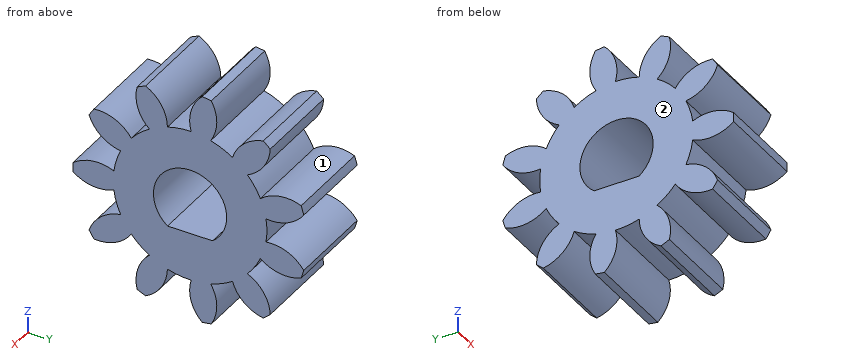
from build123d import *

# Parameters (mm, degrees)
BASPROSKE_W        = 6.35
BASPROSKE_H        = 8.255
TOOTHCUT_DEPTH     = 14.289565456
TEETHCUTS_COUNT    = 11
TEETHCUTS_ANGLE    = 327.272727273
BORSKE_R           = 1.5875
BORE_DEPTH         = 50.8000508
SKETCH1_R          = 1.5875
CUT_EXTRUDE1_DEPTH = 14.262197482


with BuildPart() as part:
    # BasProSke → Base-Revolve (revolve)
    with BuildSketch(Plane(origin=(0, 0, 0), x_dir=(1, 0, 0), z_dir=(0, 1, 0)), mode=Mode.PRIVATE) as base_revolve_sk:
        with Locations((3.175, 4.1275)):
            Rectangle(BASPROSKE_W, BASPROSKE_H)
    revolve(base_revolve_sk.sketch.rotate(Axis((-10, 0, 0), (1, 0, 0)), 180), axis=Axis((-10, 0, 0), (1, 0, 0)))

    # TooCutSke → ToothCut (cut, through all)
    with BuildSketch(Plane(origin=(0, 0, 0), x_dir=(0, 0, -1), z_dir=(1, 0, 0))):
        with BuildLine():
            ThreePointArc((0.844285256, 5.34391677), (0, 5.4102), (-0.844285256, 5.34391677))
            ThreePointArc((-0.844285256, 5.34391677), (-1.061642965, 6.854251062), (-2.040080862, 8.025153845))
            ThreePointArc((-2.040080862, 8.025153845), (0, 8.2804), (2.040080862, 8.025153845))
            ThreePointArc((2.040080862, 8.025153845), (1.061642965, 6.854251062), (0.844285256, 5.34391677))
        make_face()
    toothcut = extrude(amount=TOOTHCUT_DEPTH, mode=Mode.SUBTRACT)

    # TeethCuts: ToothCut ×11 about axis
    teethcuts_axis = Axis((-10, 0, 0), (1, 0, 0))
    for i in range(1, TEETHCUTS_COUNT):
        add(toothcut.rotate(teethcuts_axis, i * TEETHCUTS_ANGLE / (TEETHCUTS_COUNT - 1)), mode=Mode.SUBTRACT)

    # BorSke → Bore (cut, symmetric)
    with BuildSketch(Plane(origin=(0, 0, 0), x_dir=(0, 0, -1), z_dir=(1, 0, 0))):
        with Locations(Location((0, 0, 0), (0, 0, 180))):
            Circle(BORSKE_R)
    extrude(amount=BORE_DEPTH, both=True, mode=Mode.SUBTRACT)

    # Sketch1 → Cut-Extrude1 (cut, through all)
    with BuildSketch(Plane(origin=(6.35, 0, 0), x_dir=(0, 0, -1), z_dir=(1, 0, 0))):
        with BuildLine():
            Line((2.033379293, -1.5875), (2.033379293, 1.5875))
            ThreePointArc((2.033379293, 1.5875), (-2.5796875, 0), (2.033379293, -1.5875))
        make_face()
        Circle(SKETCH1_R, mode=Mode.SUBTRACT)
    extrude(amount=-CUT_EXTRUDE1_DEPTH, mode=Mode.SUBTRACT)


solid = part.part
Geometry: final body of the model. Coordinates: model frame, mm. Face numbers are marked on the shaded views. Round coordinates to 2 decimals unless told otherwise and drop trailing zeros. Order: outer loops, then holes, each group sorted by start corner. A loop starts at its lowest first (then second) coordinate and runs counter-clockwise, first axis right, second up. Notation, with made-up numbers: (17.5, 25) -> (47.5, 25) arc R10 ccw to (47.5, 44) -> close; hole circle Ø9 at (35.25, 63). An arc over 180 degrees is marked (long way). Put each result on its own line as item: value. Start each with the question number.
Q1. Section A-A on z = 0. Return the cut outline in (x, y) (3 decimals), and give its area (3 significant figures).
Q2. Pull-direction query (Y, two-part tool) for the marked faces 1 and 2; classes: +Y half, -Y half, draft (parallel to the pull), parting line (faces both ways), or undercut.
Q3. Section C-C on y = -0.5. Return the cut outline in (x, z).
Q4. Line query: probe 1 along Y at (x, z) = (2.75, 0) (3 decimals); probe 2 along Y at (x, z) = (1, -6.25); probe 3 along Z at (x, y) = (2, -6.5). Output: solid intervals per line, ascending.
Q5. Section B-B on y = -6.5. Return the cut outline in (x, z).
Q6. First-contact query: pin 1 (3 mm diameter, centred on x = 1, z = 5.5, fed in from -Y); pin 2 (3 mm diameter, centred on x = 2, y = 4.5, fed in from +Z); pin 3 (2 mm diameter, centred on x = 4.5, y = -5.5, fed in from +Z). Flat tips, straight axial feed; report the tip coordinate or a pass-through.
Ans:
1. outline: (0, -8.255) -> (6.35, -8.255) -> (6.35, -2.58) -> (0, -2.58) -> close; (0, 2.58) -> (6.35, 2.58) -> (6.35, 5.41) -> (0, 5.41) -> close
1. area: 54.0 mm2
2. face 1: undercut
2. face 2: draft
3. outline: (0, -5.39) -> (6.35, -5.39) -> (6.35, -2.03) -> (0, -2.03) -> close; (0, 2.53) -> (6.35, 2.53) -> (6.35, 5.39) -> (0, 5.39) -> close
4. probe 1: y = -8.255 to -2.58, 2.58 to 5.41
4. probe 2: y = -3.77 to -1.82, -0.03 to 1.85, 4.52 to 5.39
4. probe 3: z = -4.75 to -3.16, -0.94 to 0.94, 3.16 to 4.75
5. outline: (0, -4.75) -> (6.35, -4.75) -> (6.35, -3.16) -> (0, -3.16) -> close; (0, -0.94) -> (6.35, -0.94) -> (6.35, 0.94) -> (0, 0.94) -> close; (0, 3.16) -> (6.35, 3.16) -> (6.35, 4.75) -> (0, 4.75) -> close
6. pin 1: stops at y = -7.11
6. pin 2: stops at z = 6.45
6. pin 3: stops at z = 4.75
